CAD build for the part. Positions are in the model's coordinates, mm. Face numbers are marked on the shaded views. A direction names the side the tool comes from. Give positions to 0.01 mm unless a question says otherwise; leave off trailing zeros. Order: outer loops, then holes, each group sorted by start corner. A loop starts at its lowest first (then second) coordinate and runs counter-clockwise, first axis right, second up. Notation, with made-up numbers: (26.25, 21.25) -> (32.25, 21.25) arc R28 ccw to (32.25, 57.25) -> close; hole circle Ø5 at (-5.75, 16.5). An arc over 180 degrees is marked (long way). Use one line per item in the form item = value. Start each with the question number.
1) Drop flat-ended pins along their axis: P1, Ø6, axis at x = -0.5, y = 9, coming from the -Z side; P2, Ø3, axis at x = -0.5, z = 62, coming from the +Y side; P3, Ø0.9, axis at x = 15, y = 15, coming from the +Z side; P4, Ø3, axis at x = -4, y = 6.5, coming from the +Z side. Give the stop position or say it passes through.
2) Cut at D-D, the plane x = 3.5. Give the cut face in (y, z).
3) Cut at C-C, the plane z = 16.5. Give the cut face in (x, y), and give its area (3 significant figures).
4) Tool access for the marked faces 1 and 2: list every direction of +Z, -Z, +X, -X, +Y, -Y with a clear straight run to the whole face (end or side of a thin tool).
5) Cut at A-A, the plane x = 15.5. Give the cut face in (y, z).
6) Probe line 1 (Y direction, x = -15.5, z = 44.8); line 2 (Y direction, x = -15, z = 45); line 3 (Z direction, x = -15, y = -13.5). List the from-to ranges inside material, lowest first.
from build123d import *

# Parameters (mm, degrees)
SKETCH_W     = 42
SKETCH_H     = 42
PAD_DEPTH    = 47.5
SKETCH001_R  = 1.5
POCKET_DEPTH = 4.5
SKETCH002_R  = 11
PAD001_DEPTH = 2
PAD002_DEPTH = 22
CHAMFER_SIZE = 4


with BuildPart() as part:
    # Sketch → Pad (new body)
    with BuildSketch(Plane.XY):
        Rectangle(SKETCH_W, SKETCH_H)
    extrude(amount=PAD_DEPTH)

    # Sketch001 → Pocket (cut)
    with BuildSketch(Plane.XY.offset(47.5)):
        with Locations((-15.5, 15.5)):
            Circle(SKETCH001_R)
        with Locations((15.5, 15.5)):
            Circle(SKETCH001_R)
        with Locations((-15.5, -15.5)):
            Circle(SKETCH001_R)
        with Locations((15.5, -15.5)):
            Circle(SKETCH001_R)
    extrude(amount=-POCKET_DEPTH, mode=Mode.SUBTRACT)

    # Sketch002 → Pad001 (new body)
    with BuildSketch(Plane.XY.offset(47.5)):
        Circle(SKETCH002_R)
    extrude(amount=PAD001_DEPTH)

    # Sketch003 → Pad002 (new body)
    with BuildSketch(Plane.XY.offset(49.5)):
        with BuildLine():
            Line((-2, 1.5), (2, 1.5))
            ThreePointArc((-2, 1.5), (0, -2.5), (2, 1.5))
        make_face()
    extrude(amount=PAD002_DEPTH)

    # Chamfer
    chamfer_edges = [part.edges().sort_by_distance(p)[0] for p in [
        (-21, -21, 23.75),
        (21, -21, 23.75),
        (21, 21, 23.75),
        (-21, 21, 23.75),
    ]]
    chamfer(chamfer_edges, length=CHAMFER_SIZE)


solid = part.part
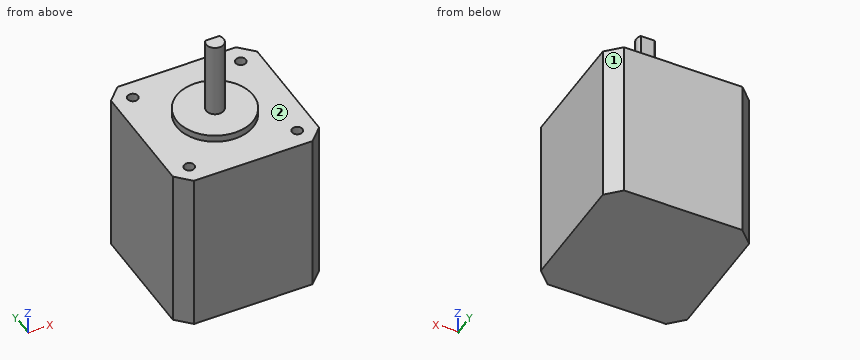
Result:
q1.P1 = 0
q1.P2 = 1.5
q1.P3 = 43
q1.P4 = 49.5
q2.outline = (-21, 0) -> (21, 0) -> (21, 47.5) -> (10.43, 47.5) -> (10.43, 49.5) -> (-10.43, 49.5) -> (-10.43, 47.5) -> (-21, 47.5) -> close
q3.outline = (-21, -17) -> (-17, -21) -> (17, -21) -> (21, -17) -> (21, 17) -> (17, 21) -> (-17, 21) -> (-21, 17) -> close
q3.area = 1,730 mm²
q4.face_1 = +Z, -Z, +X, +Y
q4.face_2 = +Z
q5.outline = (-21, 0) -> (21, 0) -> (21, 47.5) -> (17, 47.5) -> (17, 43) -> (14, 43) -> (14, 47.5) -> (-14, 47.5) -> (-14, 43) -> (-17, 43) -> (-17, 47.5) -> (-21, 47.5) -> close
q6.line_1 = -21 to -17, -14 to 14, 17 to 21
q6.line_2 = -21 to -16.91, -14.09 to 14.09, 16.91 to 21
q6.line_3 = 0 to 47.5
